Read the model definition and answer for the solid it produces. Units are mm, in the model's axes. A direction names the side the tool comes from. Round coordinates to 2 decimals unless told otherwise and drop trailing zeros. Order: outer loops, then holes, each group sorted by start corner. A loop starts at its lowest first (then second) coordinate and runs counter-clockwise, first axis right, second up. Notation, with made-up numbers: (-33, 50.5) -> (-22, 50.5) arc R35 cw to (-22, 85.5) -> close; hole circle Ø11 at (11, 44). An arc over 180 degrees is marked (long way). Answer as a JSON object with one key per item and string values. Group by question number.
Item 1: Consider probe 1 along Y at (x, z) = (0, 32); probe 2 along X at (y, z) = (36, 38.5); probe 3 along X at (y, z) = (43, 8.5). Determine where each line is inside the solid, lowest interval first. Write a range as from..to.
Item 2: Section B-B, the plane y = 0 is taken. Write down the section's boundary in (x, z).
Item 3: For faces 1 (the flat face through (-16.97, -61.24, 30.42)), 2 (the flat face through (-61.515, -15.924, 30.42)), 3 (the flat face through (-36.89, 51.74, 30.42)), 4 (the cylindrical face through (-67.6, 12, 0.5)), 5 (the flat face through (-63.251, -6.076, 30.42)), determine the directions among +Z, -Z, +X, -X, +Y, -Y from which every point of the face is accessible in a straight line to the end or side of a thin tool.
Item 4: Given P1, Ø6, axis at x = -7.5, z = 53, coming from the +Y side; P2, Ø3.5, axis at y = -65, z = 34, coming from the +X side; P3, Ø1, axis at x = 27.5, z = 42, coming from the +Y side; P4, Ø18, axis at x = 0, y = 0, coming from the -Z side, each flat-ended and moving along its own axis, determine where each tip first touches the part or whether it passes through.
Item 5: The mould has two halves that part along X. Classify faces 6 (the cylindrical face through (-61.93, -31.02, 29.58)), 7 (the flat face through (36.89, 51.74, 30.42)), 8 (the flat face through (60.636, -34.976, 30.378)): pulls with the +X half, pulls with the -X half, needs draft (parallel to the pull), parting line crosses it, or undercut.
Item 6: Section A-A, the plane x = 0 is taken. Write down the section's boundary in (y, z).
Item 7: Section C-C, the plane y = 23.5 is taken. Write down the section's boundary in (x, z).
from build123d import *

# Parameters (mm, degrees)
SKETCH2_R                = 60
BOSS_EXTRUDE1_DEPTH      = 60
SKETCH3_W                = 10
SKETCH3_H                = 10.47851478
BOSS_EXTRUDE2_DEPTH      = 60
FILLET2_R                = 3
CIRPATTERN1_COUNT        = 18
FILLET2_OF_CIRPATTERN1_R = 3
SKETCH4_R                = 10
CUT_EXTRUDE1_DEPTH       = 60


with BuildPart() as part:
    # Sketch2 → Boss-Extrude1 (new body)
    with BuildSketch(Plane.XY):
        Circle(SKETCH2_R)
    extrude(amount=BOSS_EXTRUDE1_DEPTH)

    # Sketch3 → Boss-Extrude2 (add)
    with BuildSketch(Plane.XY.offset(60)):
        with Locations((0, 64.76074261)):
            Rectangle(SKETCH3_W, SKETCH3_H)
    boss_extrude2 = extrude(amount=-BOSS_EXTRUDE2_DEPTH)

    # Fillet2
    fillet2_edges = [part.edges().sort_by_distance(p)[0] for p in [
        (5, 70, 30),
        (0, 70, 0),
        (-5, 70, 30),
        (0, 70, 60),
    ]]
    fillet(fillet2_edges, radius=FILLET2_R)

    # CirPattern1: Boss-Extrude2 ×18 about axis
    cirpattern1_axis = Axis((0, 0, 0), (0, 0, 1))
    for i in range(1, CIRPATTERN1_COUNT):
        add(boss_extrude2.rotate(cirpattern1_axis, i * 360 / CIRPATTERN1_COUNT))

    # Fillet2 of CirPattern1
    fillet2_of_cirpattern1_edges = [part.edges().sort_by_distance(p)[0] for p in [
        (-19.242946929, 67.488584172, 30),
        (-23.941410033, 65.778483455, 0),
        (-28.639873137, 64.068382738, 30),
        (-23.941410033, 65.778483455, 60),
        (-41.164910462, 56.837049067, 30),
        (-44.995132678, 53.623111018, 0),
        (-48.825354894, 50.40917297, 30),
        (-44.995132678, 53.623111018, 60),
        (-58.121778265, 39.330127019, 30),
        (-60.621778265, 35, 0),
        (-63.121778265, 30.669872981, 30),
        (-60.621778265, 35, 60),
        (-68.068301823, 17.079411202, 30),
        (-68.936542711, 12.155372437, 0),
        (-69.804783599, 7.231333672, 30),
        (-68.936542711, 12.155372437, 60),
        (-69.804783599, -7.231333672, 30),
        (-68.936542711, -12.155372437, 0),
        (-68.068301823, -17.079411202, 30),
        (-68.936542711, -12.155372437, 60),
        (-63.121778265, -30.669872981, 30),
        (-60.621778265, -35, 0),
        (-58.121778265, -39.330127019, 30),
        (-60.621778265, -35, 60),
        (-48.825354894, -50.40917297, 30),
        (-44.995132678, -53.623111018, 0),
        (-41.164910462, -56.837049067, 30),
        (-44.995132678, -53.623111018, 60),
        (-28.639873137, -64.068382738, 30),
        (-23.941410033, -65.778483455, 0),
        (-19.242946929, -67.488584172, 30),
        (-23.941410033, -65.778483455, 60),
        (-5, -70, 30),
        (0, -70, 0),
        (5, -70, 30),
        (0, -70, 60),
        (19.242946929, -67.488584172, 30),
        (23.941410033, -65.778483455, 0),
        (28.639873137, -64.068382738, 30),
        (23.941410033, -65.778483455, 60),
        (41.164910462, -56.837049067, 30),
        (44.995132678, -53.623111018, 0),
        (48.825354894, -50.40917297, 30),
        (44.995132678, -53.623111018, 60),
        (58.121778265, -39.330127019, 30),
        (60.621778265, -35, 0),
        (63.121778265, -30.669872981, 30),
        (60.621778265, -35, 60),
        (68.068301823, -17.079411202, 30),
        (68.936542711, -12.155372437, 0),
        (69.804783599, -7.231333672, 30),
        (68.936542711, -12.155372437, 60),
        (69.804783599, 7.231333672, 30),
        (68.936542711, 12.155372437, 0),
        (68.068301823, 17.079411202, 30),
        (68.936542711, 12.155372437, 60),
        (63.121778265, 30.669872981, 30),
        (60.621778265, 35, 0),
        (58.121778265, 39.330127019, 30),
        (60.621778265, 35, 60),
        (48.825354894, 50.40917297, 30),
        (44.995132678, 53.623111018, 0),
        (41.164910462, 56.837049067, 30),
        (44.995132678, 53.623111018, 60),
        (28.639873137, 64.068382738, 30),
        (23.941410033, 65.778483455, 0),
        (19.242946929, 67.488584172, 30),
        (23.941410033, 65.778483455, 60),
    ]]
    fillet(fillet2_of_cirpattern1_edges, radius=FILLET2_OF_CIRPATTERN1_R)

    # Sketch4 → Cut-Extrude1 (cut)
    with BuildSketch(Plane.XY.offset(60)):
        Circle(SKETCH4_R)
    extrude(amount=-CUT_EXTRUDE1_DEPTH, mode=Mode.SUBTRACT)


solid = part.part
Values found:
{
 "1": {"probe 1": "-70..-10, 10..70", "probe 2": "-60.04..-52.35, -48..48, 52.35..60.04", "probe 3": "-42.61..42.61"},
 "2": {"outline": "(-60, 0) -> (-10, 0) -> (-10, 60) -> (-60, 60) -> close; (10, 0) -> (60, 0) -> (60, 60) -> (10, 60) -> close"},
 "3": {"face 1": "+Z, -Z, -Y", "face 2": "+Z, -Z", "face 3": "+Z, -Z, +Y", "face 4": "-Z, -X, +Y", "face 5": "+Z, -Z, -X"},
 "4": {"P1": "y = 68.66", "P2": "x = 27.63", "P3": "y = 64.31", "P4": "through"},
 "5": {"face 6": "pulls with the -X half", "face 7": "undercut", "face 8": "pulls with the +X half"},
 "6": {"outline": "(-70, 3) arc R3 ccw to (-67, 0) -> (-10, 0) -> (-10, 60) -> (-67, 60) arc R3 ccw to (-70, 57) -> close; (10, 0) -> (67, 0) arc R3 ccw to (70, 3) -> (70, 57) arc R3 ccw to (67, 60) -> (10, 60) -> close"},
 "7": {"outline": "(-55.21, 0) -> (55.21, 0) -> (55.21, 60) -> (-55.21, 60) -> close"}
}
